Part print with two shaded views. Sizes in mm from the minimum x, y, z corner. A direction names the side the tool comes from. Coordinates: 2 decimals unless noted, no trailing zeros. Write each loop counter-clockwise with the first axis right and the second up, starting at its lowest first coordinate (ties: lowest second). Pieces come first, ordered by that corner, then holes. Notation, with made-up numbers: (75, 10.5) - (93, 10.5) arc R22 cw to (93, 46.5) - close; hole circle Ø7 at (-11, 23.5). An arc over 180 degrees is marked (long way). One line per question, with ' | ' between items. Start each with the question number.
1. Band-saw the part on D-D, the plane y = 8. Write the cut outline in (x, z), then the cut area to 3 significant figures.
2. Band-saw the part on A-A, the plane y = 24. Write the cut outline in (x, z), then the cut area to 3 significant figures.
3. Band-saw the part on C-C, the plane x = 20.5. Write the cut outline in (y, z), then the cut area to 3 significant figures.
4. Band-saw the part on B-B, the plane z = 3.25. Write the cut outline in (x, y), then the cut area to 3 significant figures.
5. Which spindle directions (+Z, -Z, +X, -X, +Y, -Y) get a long thin tool onto all of the face, cutting with end or side? Do the marked faces 1, 2 and 3. Say none if no direction does.
6. Flat gauge pins, fed straight in: P1, Ø1.5, axis at x = 26.5, z = 4, coming from the +Y side (3 decimals); P2, Ø2, axis at x = 34.5, z = 3, coming from the +Y side; P3, Ø2.5, axis at x = 21.5, z = 2, coming from the +Y side. Where does each tip first touch, or does it go through?
7. Probe line 1 (Y direction, x = 23.5, z = 1.5); line 2 (X direction, y = 21.5, z = 4.5); line 3 (Y direction, x = 10.5, z = 6). List the from-to ranges inside material, lowest first.
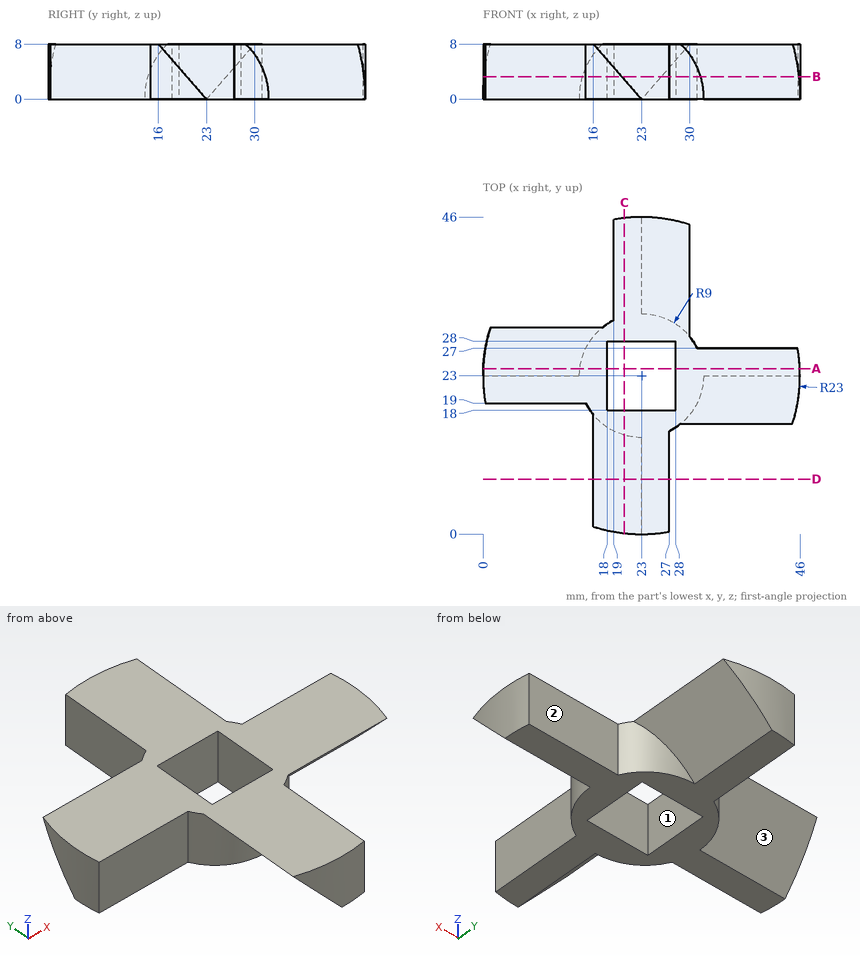
Filled in:
1) outline: (16, 8) - (23, 0) - (27, 0) - (27, 8) - close | area: 60.0 mm²
2) outline: (0.02, 1.14) - (14.06, 1.14) - (14.06, 0) - (18, 0) - (18, 8) - (0.02, 8) - close; (28, 0) - (45.98, 0) - (45.98, 8) - (28, 8) - close | area: 272 mm²
3) outline: (0.14, 2.86) - (14.35, 2.86) - (14.35, 0) - (18, 0) - (18, 8) - (0.14, 8) - close; (28, 0) - (45.86, 0) - (45.86, 8) - (28, 8) - close | area: 245 mm²
4) outline: (0.18, 25.84) arc R23 ccw to (0.35, 19) - (14.94, 19) arc R9 ccw to (20.16, 14.46) - (20.16, 0.18) arc R23 ccw to (27, 0.35) - (27, 14.94) arc R9 ccw to (31.54, 20.16) - (45.82, 20.16) arc R23 ccw to (45.65, 27) - (31.06, 27) arc R9 ccw to (25.84, 31.54) - (25.84, 45.82) arc R23 ccw to (19, 45.65) - (19, 31.06) arc R9 ccw to (14.46, 25.84) - close; hole (18, 18) - (28, 18) - (28, 28) - (18, 28) - close | area: 542 mm²
5) face 1: +Z, -Z | face 2: +Z, -Z, +X, +Y | face 3: -Z, -X, +Y
6) P1: stops at y = 45.835 | P2: stops at y = 27 | P3: stops at y = 46
7) line 1: y = 0.01 to 18, 28 to 45.99 | line 2: x = 0.05 to 18, 28 to 45.95 | line 3: y = 19 to 28.25
